from build123d import *

# Parameters (mm, degrees)
SKETCH1_W           = 80
SKETCH1_H           = 12.7
BOSS_EXTRUDE1_DEPTH = 12.7
SKETCH2_R           = 5
CUT_EXTRUDE1_DEPTH  = 13.7
SKETCH3_R           = 2.15
SKETCH3_R_2         = 2.65
CUT_EXTRUDE2_DEPTH  = 13.7
BOSS_EXTRUDE2_START = -1.25
SKETCH4_W           = 0.5
SKETCH4_H           = 20
BOSS_EXTRUDE2_DEPTH = 10


with BuildPart() as part:
    # Sketch1 → Boss-Extrude1 (new body)
    with BuildSketch(Plane(origin=(0, 0, 0), x_dir=(0, 0, -1), z_dir=(1, 0, 0))):
        Rectangle(SKETCH1_W, SKETCH1_H)
    extrude(amount=BOSS_EXTRUDE1_DEPTH)

    # Sketch2 → Cut-Extrude1 (cut, through all)
    with BuildSketch(Plane(origin=(0, 6.35, 0), x_dir=(1, 0, 0), z_dir=(0, 1, 0))):
        with Locations((6.35, -3.75)):
            Circle(SKETCH2_R)
        with Locations((6.35, 3.75)):
            Circle(SKETCH2_R)
    extrude(amount=-CUT_EXTRUDE1_DEPTH, mode=Mode.SUBTRACT)

    # Sketch3 → Cut-Extrude2 (cut, through all)
    with BuildSketch(Plane(origin=(12.7, 0, 0), x_dir=(0, 0, -1), z_dir=(1, 0, 0))):
        with Locations((-35, 0)):
            Circle(SKETCH3_R)
        with Locations((-20, 0)):
            Circle(SKETCH3_R)
        with Locations((20, 0)):
            Circle(SKETCH3_R_2)
        with Locations((35, 0)):
            Circle(SKETCH3_R_2)
    extrude(amount=-CUT_EXTRUDE2_DEPTH, mode=Mode.SUBTRACT)

    # Sketch4 → Boss-Extrude2 (add)
    with BuildSketch(Plane(origin=(0, 6.35, 0), x_dir=(1, 0, 0), z_dir=(0, 1, 0)).offset(BOSS_EXTRUDE2_START)):
        with Locations((-0.25, 0)):
            Rectangle(SKETCH4_W, SKETCH4_H)
        with Locations((12.95, 0)):
            Rectangle(SKETCH4_W, SKETCH4_H)
    extrude(amount=-BOSS_EXTRUDE2_DEPTH)


solid = part.part
Design review of the part built by this model. Coordinates are the model's own, in mm. Round coordinates to 2 decimals unless told otherwise and drop trailing zeros. Loops run counter-clockwise (first coordinate to the right, second up) from the corner with the lowest first, then second, coordinate; pieces in that order, holes last. Notation, with made-up numbers: M 49.5,40 L 92.5,40 A27 ccw 92.5,70 Z; hole C 5,9 d10. An arc over 180 degrees is marked long. Answer as a JSON object with one key per item and string values.
Item 1: We need section C-C on y = -1.25. State how many separate pieces and enclosed holes the cut face has, and give its area (3 significant figures).
Answer sheet:
{"separate pieces": "5", "enclosed holes": "1", "area": "683 mm^2"}
Item 2: The part is to be moulded in two halves that separate along Y. For faces 1 (the cylindrical face through (6.181, 0.089, 8.747)), 2 (the flat face through (10.5, -6.35, 0.6)), 3 (the cylindrical face through (6.44, 0.09, 22.15)), say which applies: pulls with the +Y half, pulls with the -Y half, needs draft (parallel to the pull), parting line crosses it, or undercut.
Answer sheet:
{"face 1": "needs draft", "face 2": "pulls with the -Y half", "face 3": "undercut"}
Item 3: We need section B-B on z = 35. Give the boundary of the cut face in (x, y).
Answer sheet:
{"outline": "M 0,-6.35 L 12.7,-6.35 L 12.7,-2.15 L 0,-2.15 Z; M 0,2.15 L 12.7,2.15 L 12.7,6.35 L 0,6.35 Z"}
Item 4: Clearance check with flat-ended pins moving along their axes: P1, Ø0.6, axis at x = -0.5, y = 1.5, coming from the -Z side; P2, Ø7, axis at y = 0, z = -20, coming from the -X side; P3, Ø4, axis at x = 5, z = -1.5, coming from the +Y side; P4, Ø0.6, axis at x = -0.5, z = -0.5, coming from the +Y side. State where each tip first meets the part, or that it passes through.
Answer sheet:
{"P1": "stops at z = -10", "P2": "stops at x = 0", "P3": "passes through", "P4": "stops at y = 5.1"}
Item 5: We need section D-D on y = 4.25. Give the boundary of the cut face in (x, z), and give its area (3 significant figures).
Answer sheet:
{"outline": "M -0.5,-10 L 0,-10 L 0,-40 L 12.7,-40 L 12.7,-10 L 13.2,-10 L 13.2,10 L 12.7,10 L 12.7,40 L 0,40 L 0,10 L -0.5,10 Z; hole M 3.04,0 A5 ccw long 9.66,0 A5 ccw long Z", "area": "890 mm^2"}
Item 6: We need section A-A on x = 6.35. Give the boundary of the cut face in (y, z).
Answer sheet:
{"outline": "M -6.35,-40 L 6.35,-40 L 6.35,-8.75 L -6.35,-8.75 Z; M -6.35,8.75 L 6.35,8.75 L 6.35,40 L -6.35,40 Z; hole C 0,-35 d5.3; hole C 0,-20 d5.3; hole C 0,20 d4.3; hole C 0,35 d4.3"}
Item 7: Wall thickness on L1, parallel to Y at x = 5.75, z = 35; L2, parallel to Y at x = 11, z = -20; L3, parallel to Z at x = 9.5, y = 1.5: over which ranges is each line inside the solid? List them lowest first. Write a range as from..to.
Answer sheet:
{"L1": "y = -6.35..-2.15, 2.15..6.35", "L2": "y = -6.35..-2.65, 2.65..6.35", "L3": "z = -40..-37.18, -32.82..-22.18, -17.82..-7.63, 7.63..18.46, 21.54..33.46, 36.54..40"}
